Input: part model. Units: mm. Frame: model coordinates. A direction names the side the tool comes from. Give positions to 0.01 mm unless a question says otherwise; leave off trailing zeros. Loops run counter-clockwise (first coordinate to the right, second up) from the corner with the lowest first, then second, coordinate; pieces in that order, holes last. Notation, with made-up numbers: M -16,38 L 6,38 A12 ccw 6,42 Z; hole C 7,46.25 d3. An arc over 180 degrees is marked long. One line per item, written item: value. Start each with the question number.
(1) Section A-A on y = -5. Output: boundary loops of the cut face in (x, z).
(2) Pull-direction query (Z, two-part tool) for faces 1 (the cylindrical face through (-0.49, 112.03, 139.99)), 2 (the flat face through (0.49, 74.886, 3.494)), 3 (the cylindrical face through (32.594, -27.719, -4.512)), 4 (the flat face through (-0.49, 93.42, 78.95)); classes: released by +Z, released by -Z, zero draft, split by the parting line, or undercut.
(3) Pin query (flat end, axial travel): P1, Ø2.5, axis at x = 20, y = 64.4, coming from the +Z side; P2, Ø7, axis at x = -20, z = 162.9, coming from the -Y side; P3, Ø1.5, axis at x = 24, y = -12, coming from the +Z side. Return the tip coordinate at first contact, or that it passes through.
(4) Section C-C on y = 43. Output: boundary loops of the cut face in (x, z), plus the area to 3 significant figures.
(5) Section B-B on z = 156. Output: boundary loops of the cut face in (x, y).
(6) Access query for faces 5 (the cylindrical face through (-0.49, 82.756, 16.268)), 6 (the flat face through (0, 112.5, 204)), 7 (the flat face through (0, 13, 0)). Directions: +Z, -Z, +X, -X, +Y, -Y. A direction counts if a zero-diameter tool reaches every point of the face in a straight line with its end or side. Return the directions, or none.
(7) Ray query, line 1 along X through (y, z) = (102.4, 274); line 2 along X through (y, z) = (116.5, 227.9); line 3 along Y through (x, z) = (0, 271). Return the intervals inside material, ascending. Write a range as from..to.
```python
from build123d import *

# Parameters (mm, degrees)
SKETCH3_W           = 70
SKETCH3_H           = 8.9
SKETCH4_R           = 12.3
BOSS_EXTRUDE1_DEPTH = 4
FILLET1_R           = 10
FILLET2_R           = 40
FILLET3_R           = 8
FILLET4_R           = 40
FILLET5_R           = 5
CUT_EXTRUDE1_REACH  = 288.8
SKETCH5_R           = 6.5
SKETCH5_R_2         = 1.25
CUT_EXTRUDE2_REACH  = 153.4
SKETCH6_R           = 2.6
CUT_EXTRUDE3_REACH  = 288.8
SKETCH7_R           = 1.5


with BuildPart() as part:
    # Sweep1: sweep along a path in Sketch1
    with BuildLine(Plane(origin=(0, 0, 0), x_dir=(0, 0, -1), z_dir=(1, 0, 0))) as sweep1_path:
        Line((-269, 61.5), (-269, 112.5))
        Line((-269, 112.5), (-140, 112.5))
        Line((-140, 112.5), (-20, 75))
        Line((-20, 75), (0, 62))
        Line((0, 62), (0, 0))
        Line((0, 0), (0, -30))
    # Sketch3 → Sweep1 (sweep)
    with BuildSketch(Plane(origin=(0, 0, 0), x_dir=(1, 0, 0), z_dir=(0, 1, 0))):
        with Locations((0, 4.45)):
            Rectangle(SKETCH3_W, SKETCH3_H)
    sweep(path=sweep1_path.line, transition=Transition.RIGHT)

    # Sketch4 → Boss-Extrude1 (add)
    with BuildSketch(Plane.XY):
        with Locations((0, -5)):
            Circle(SKETCH4_R)
    extrude(amount=BOSS_EXTRUDE1_DEPTH)

    # Fillet1
    fillet1_edges = [part.edges().sort_by_distance(p)[0] for p in [
        (0, 66.829905793, -8.9),
        (0, 62, 0),
    ]]
    fillet(fillet1_edges, radius=FILLET1_R)

    # Fillet2
    fillet2_edges = [part.edges().sort_by_distance(p)[0] for p in [
        (0, 83.129581848, 16.176424699),
        (0, 75, 20),
    ]]
    fillet(fillet2_edges, radius=FILLET2_R)

    # Fillet3
    fillet3_edges = [part.edges().sort_by_distance(p)[0] for p in [
        (35, -30, -4.45),
        (-35, -30, -4.45),
    ]]
    fillet(fillet3_edges, radius=FILLET3_R)

    # Fillet4
    fillet4_edges = [part.edges().sort_by_distance(p)[0] for p in [
        (0, 121.4, 138.641762787),
        (0, 112.5, 140),
    ]]
    fillet(fillet4_edges, radius=FILLET4_R)

    # Fillet5
    fillet5_edges = [part.edges().sort_by_distance(p)[0] for p in [
        (0, 112.5, 269),
        (0, 121.4, 277.9),
    ]]
    fillet(fillet5_edges, radius=FILLET5_R)

    # Sketch5 → Cut-Extrude1 (cut, up to next)
    with BuildSketch(Plane.XY.offset(277.9), mode=Mode.PRIVATE) as cut_extrude1_sk1:
        with Locations((0, 87.04)):
            Circle(SKETCH5_R)
    cut_extrude1_tool1 = extrude(cut_extrude1_sk1.sketch, amount=-CUT_EXTRUDE1_REACH, mode=Mode.PRIVATE) & part.part
    add(cut_extrude1_tool1.solids().sort_by_distance((0, 87.04, 277.9))[0], mode=Mode.SUBTRACT)
    # Sketch5 → Cut-Extrude1 (cut, up to next)
    with BuildSketch(Plane.XY.offset(277.9), mode=Mode.PRIVATE) as cut_extrude1_sk2:
        with Locations((-0.2, 96.49)):
            Circle(SKETCH5_R_2)
    cut_extrude1_tool2 = extrude(cut_extrude1_sk2.sketch, amount=-CUT_EXTRUDE1_REACH, mode=Mode.PRIVATE) & part.part
    add(cut_extrude1_tool2.solids().sort_by_distance((-0.2, 96.49, 277.9))[0], mode=Mode.SUBTRACT)
    # Sketch5 → Cut-Extrude1 (cut, up to next)
    with BuildSketch(Plane.XY.offset(277.9), mode=Mode.PRIVATE) as cut_extrude1_sk3:
        with Locations((0.4, 77.59)):
            Circle(SKETCH5_R_2)
    cut_extrude1_tool3 = extrude(cut_extrude1_sk3.sketch, amount=-CUT_EXTRUDE1_REACH, mode=Mode.PRIVATE) & part.part
    add(cut_extrude1_tool3.solids().sort_by_distance((0.4, 77.59, 277.9))[0], mode=Mode.SUBTRACT)
    # Sketch5 → Cut-Extrude1 (cut, up to next)
    with BuildSketch(Plane.XY.offset(277.9), mode=Mode.PRIVATE) as cut_extrude1_sk4:
        with Locations((-9.45, 86.84)):
            Circle(SKETCH5_R_2)
    cut_extrude1_tool4 = extrude(cut_extrude1_sk4.sketch, amount=-CUT_EXTRUDE1_REACH, mode=Mode.PRIVATE) & part.part
    add(cut_extrude1_tool4.solids().sort_by_distance((-9.45, 86.84, 277.9))[0], mode=Mode.SUBTRACT)
    # Sketch5 → Cut-Extrude1 (cut, up to next)
    with BuildSketch(Plane.XY.offset(277.9), mode=Mode.PRIVATE) as cut_extrude1_sk5:
        with Locations((9.45, 87.44)):
            Circle(SKETCH5_R_2)
    cut_extrude1_tool5 = extrude(cut_extrude1_sk5.sketch, amount=-CUT_EXTRUDE1_REACH, mode=Mode.PRIVATE) & part.part
    add(cut_extrude1_tool5.solids().sort_by_distance((9.45, 87.44, 277.9))[0], mode=Mode.SUBTRACT)

    # Sketch6 → Cut-Extrude2 (cut, up to next)
    with BuildSketch(Plane(origin=(0, 121.4, 0), x_dir=(1, 0, 0), z_dir=(0, 1, 0)), mode=Mode.PRIVATE) as cut_extrude2_sk1:
        with Locations((-20, -162.9)):
            Circle(SKETCH6_R)
    cut_extrude2_tool1 = extrude(cut_extrude2_sk1.sketch, amount=-CUT_EXTRUDE2_REACH, mode=Mode.PRIVATE) & part.part
    add(cut_extrude2_tool1.solids().sort_by_distance((-20, 121.4, 162.9))[0], mode=Mode.SUBTRACT)
    # Sketch6 → Cut-Extrude2 (cut, up to next)
    with BuildSketch(Plane(origin=(0, 121.4, 0), x_dir=(1, 0, 0), z_dir=(0, 1, 0)), mode=Mode.PRIVATE) as cut_extrude2_sk2:
        with Locations((20, -162.9)):
            Circle(SKETCH6_R)
    cut_extrude2_tool2 = extrude(cut_extrude2_sk2.sketch, amount=-CUT_EXTRUDE2_REACH, mode=Mode.PRIVATE) & part.part
    add(cut_extrude2_tool2.solids().sort_by_distance((20, 121.4, 162.9))[0], mode=Mode.SUBTRACT)
    # Sketch6 → Cut-Extrude2 (cut, up to next)
    with BuildSketch(Plane(origin=(0, 121.4, 0), x_dir=(1, 0, 0), z_dir=(0, 1, 0)), mode=Mode.PRIVATE) as cut_extrude2_sk3:
        with Locations((-20, -227.9)):
            Circle(SKETCH6_R)
    cut_extrude2_tool3 = extrude(cut_extrude2_sk3.sketch, amount=-CUT_EXTRUDE2_REACH, mode=Mode.PRIVATE) & part.part
    add(cut_extrude2_tool3.solids().sort_by_distance((-20, 121.4, 227.9))[0], mode=Mode.SUBTRACT)
    # Sketch6 → Cut-Extrude2 (cut, up to next)
    with BuildSketch(Plane(origin=(0, 121.4, 0), x_dir=(1, 0, 0), z_dir=(0, 1, 0)), mode=Mode.PRIVATE) as cut_extrude2_sk4:
        with Locations((20, -227.9)):
            Circle(SKETCH6_R)
    cut_extrude2_tool4 = extrude(cut_extrude2_sk4.sketch, amount=-CUT_EXTRUDE2_REACH, mode=Mode.PRIVATE) & part.part
    add(cut_extrude2_tool4.solids().sort_by_distance((20, 121.4, 227.9))[0], mode=Mode.SUBTRACT)

    # Sketch7 → Cut-Extrude3 (cut, up to next)
    with BuildSketch(Plane.XY.offset(277.9), mode=Mode.PRIVATE) as cut_extrude3_sk1:
        with Locations((20, 102.4)):
            Circle(SKETCH7_R)
    cut_extrude3_tool1 = extrude(cut_extrude3_sk1.sketch, amount=-CUT_EXTRUDE3_REACH, mode=Mode.PRIVATE) & part.part
    add(cut_extrude3_tool1.solids().sort_by_distance((20, 102.4, 277.9))[0], mode=Mode.SUBTRACT)
    # Sketch7 → Cut-Extrude3 (cut, up to next)
    with BuildSketch(Plane.XY.offset(277.9), mode=Mode.PRIVATE) as cut_extrude3_sk2:
        with Locations((20, 64.4)):
            Circle(SKETCH7_R)
    cut_extrude3_tool2 = extrude(cut_extrude3_sk2.sketch, amount=-CUT_EXTRUDE3_REACH, mode=Mode.PRIVATE) & part.part
    add(cut_extrude3_tool2.solids().sort_by_distance((20, 64.4, 277.9))[0], mode=Mode.SUBTRACT)
    # Sketch7 → Cut-Extrude3 (cut, up to next)
    with BuildSketch(Plane.XY.offset(277.9), mode=Mode.PRIVATE) as cut_extrude3_sk3:
        with Locations((-20, 102.4)):
            Circle(SKETCH7_R)
    cut_extrude3_tool3 = extrude(cut_extrude3_sk3.sketch, amount=-CUT_EXTRUDE3_REACH, mode=Mode.PRIVATE) & part.part
    add(cut_extrude3_tool3.solids().sort_by_distance((-20, 102.4, 277.9))[0], mode=Mode.SUBTRACT)
    # Sketch7 → Cut-Extrude3 (cut, up to next)
    with BuildSketch(Plane.XY.offset(277.9), mode=Mode.PRIVATE) as cut_extrude3_sk4:
        with Locations((-20, 64.4)):
            Circle(SKETCH7_R)
    cut_extrude3_tool4 = extrude(cut_extrude3_sk4.sketch, amount=-CUT_EXTRUDE3_REACH, mode=Mode.PRIVATE) & part.part
    add(cut_extrude3_tool4.solids().sort_by_distance((-20, 64.4, 277.9))[0], mode=Mode.SUBTRACT)


solid = part.part
```
Output values:
1. outline: M -35,-8.9 L 35,-8.9 L 35,0 L 12.3,0 L 12.3,4 L -12.3,4 L -12.3,0 L -35,0 Z
2. face 1: undercut
2. face 2: released by -Z
2. face 3: zero draft
2. face 4: undercut
3. P1: stops at z = 5.62
3. P2: stops at y = 112.5
3. P3: stops at z = 0
4. outline: M -35,-8.9 L 35,-8.9 L 35,0 L -35,0 Z
4. area: 623 mm²
5. outline: M -35,112.5 L 35,112.5 L 35,121.4 L -35,121.4 Z
6. face 5: -Z, +X, -X, +Y
6. face 6: +X, -X, -Y
6. face 7: +Z
7. line 1: x = -35..-21.5, -18.5..18.5, 21.5..35
7. line 2: x = -35..-22.6, -17.4..17.4, 22.6..35
7. line 3: y = 61.5..76.41, 78.77..80.54, 93.54..95.26, 97.72..121.4
